from build123d import *

# Parameters (mm, degrees)
F0_R     = 9.953913
F2_DEPTH = 8


with BuildPart() as f2:
    # F0 (on Top) → F2 (new body)
    with BuildSketch(Plane.XY):
        with BuildLine():
            ThreePointArc((29.868933, 7.770019), (35.48766, 13.226767), (37.551685, 20.782295))
            ThreePointArc((37.551685, 20.782295), (29.148663, 34.166644), (13.442543, 32.414685))
            ThreePointArc((13.442543, 32.414685), (13.34143, 32.333237), (13.240702, 32.251313))
            ThreePointArc((13.240702, 32.251313), (10.397613, 12.432448), (29.868933, 7.770019))
        make_face()
        with Locations((22.690865, 20.782295)):
            Circle(F0_R, mode=Mode.SUBTRACT)
        with BuildLine():
            ThreePointArc((44.149149, -13.117656), (29.767923, -7.624333), (29.868933, 7.770019))
            ThreePointArc((29.868933, 7.770019), (10.397613, 12.432448), (13.240702, 32.251313))
            ThreePointArc((13.240702, 32.251313), (7.905379, -4.596433), (44.149149, -13.117656))
        make_face()
    extrude(amount=F2_DEPTH)


solid = f2.part
Build history of the part. All positions in model axes, mm. Coordinates: 2 decimals unless noted, no trailing zeros. Order: outer loops, then holes, each group sorted by start corner. A loop starts at its lowest first (then second) coordinate and runs counter-clockwise, first axis right, second up. Notation, with made-up numbers: (21.5, -12) - (74.5, -12) arc R10 cw to (74.5, -2) - close; hole circle Ø5 at (-39.5, -21). An arc over 180 degrees is marked (long way). Write item = value, one per line. Start each with the question number.
1) Wall check: line 1 along Y through (x, z) = (26, 2.75); line 2 along X through (y, z) = (18.5, 7.75); line 3 along X through (y, z) = (24.5, 6.75). Give the ranges that are in metal, low to high. Write a range as from..to.
2) Flat gauge pins, fed straight in: pin 1 Ø12 at (x, y) = (22.69, 20.78) entering from +Z; pin 2 Ø1.5 at (y, z) = (0.5, 3) entering from -X. Where does each tip first touch, or does it go through?
3) Saw through at A-A on x = 18.5. Write the cut outline in (y, z).
4) Saw through at B-B on z = 6.75. Write the cut outline in (x, y), then the cut area to 3 significant figures.
5) Saw through at C-C on x = 24.5. Write the cut outline in (y, z), then the cut area to 3 significant figures.
6) Saw through at D-D on y = 1.5. Write the cut outline in (x, z).
7) Two-plate mould, pull along Y, no slides. Class faces 1 (the face through (7.59, -4.12, 3.94)), 2 (the face through (28, 29.2, 3.9)), 3 (the face through (19, 10, 0)): pulls with the +Y half, pulls with the -Y half, needs draft (parallel to the pull), parting line crosses it, or undercut.
From the geometry:
q1.line_1 = -16.24..11.39, 30.17..35.27
q1.line_2 = 4.19..13, 32.38..37.38
q1.line_3 = 6.7..13.46, 31.92..37.08
q2.pin_1 = through
q2.pin_2 = 4.87
q3.outline = (-13.8, 0) - (11.75, 0) - (11.75, 8) - (-13.8, 8) - close; (29.81, 0) - (35.04, 0) - (35.04, 8) - (29.81, 8) - close
q4.outline = (13.24, 32.25) arc R27.55 ccw to (44.15, -13.12) arc R13.51 cw to (29.87, 7.77) arc R14.86 ccw to (37.55, 20.78) arc R14.86 ccw to (13.44, 32.41) arc R27.54 ccw to start; hole circle Ø19.91 at (22.69, 20.78)
q4.area = 974 mm^2
q5.outline = (-15.94, 0) - (10.99, 0) - (10.99, 8) - (-15.94, 8) - close; (30.57, 0) - (35.53, 0) - (35.53, 8) - (30.57, 8) - close
q5.area = 255 mm^2
q6.outline = (4.78, 0) - (27.49, 0) - (27.49, 8) - (4.78, 8) - close
q7.face_1 = parting line crosses it
q7.face_2 = undercut
q7.face_3 = needs draft
